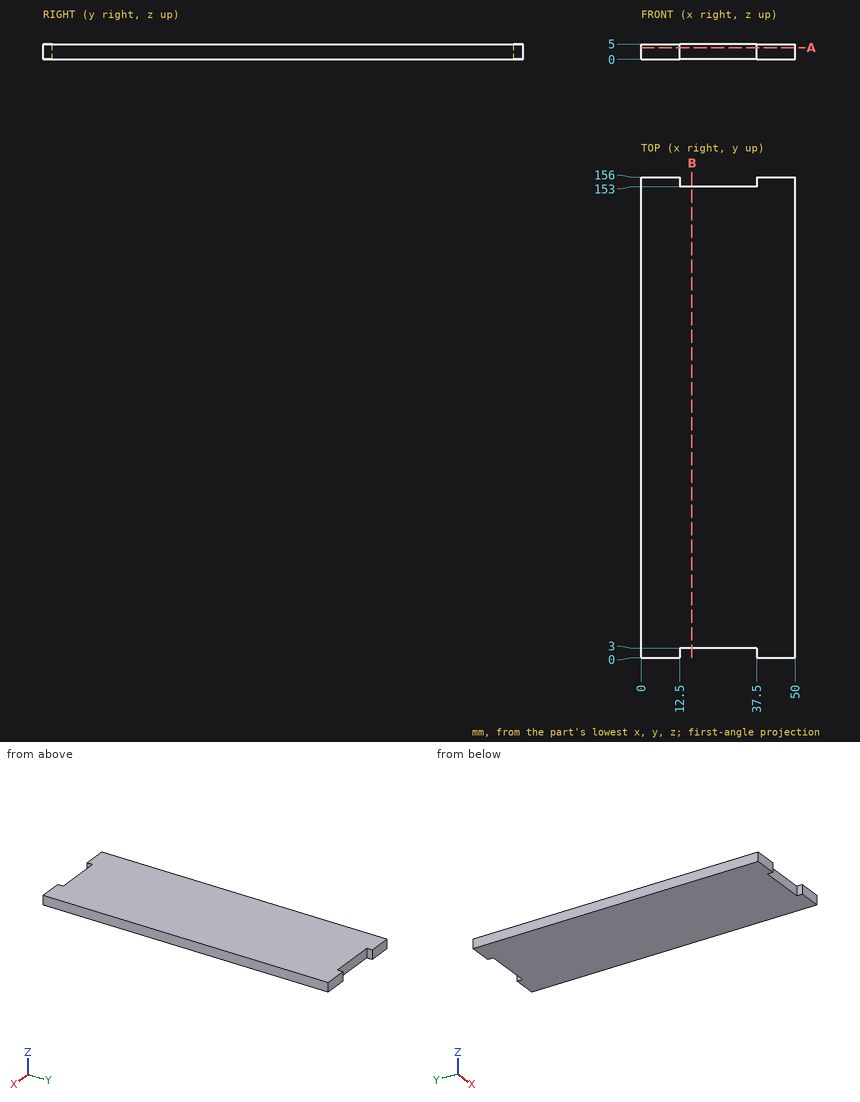
Study the drawing (mm; zero at the part's minimum x, y, z) and answer. Coordinates: 2 decimals unless noted, no trailing zeros. Write each loop counter-clockwise with the first axis right and the second up, starting at its lowest first coordinate (ties: lowest second). Pieces come first, ordered by that corner, then holes. Notation, with made-up numbers: (72, 30.25) - (93, 30.25) arc R12 ccw to (93, 40.25) - close; hole circle Ø6 at (83.25, 30). An arc over 180 degrees is marked (long way). Answer as a JSON object with one key per item and string values. Group by question number.
1. Consider L1, parallel to Y at x = 17, z = 1.2. Determine where the line is inside the solid, lowest interval first. Write a range as [from, to].
2. A cutting plane is placed at A-A (z = 3.85). Determine the outline of the cut face in (x, y).
3. A cutting plane is placed at B-B (x = 16.5). Determine the outline of the cut face in (y, z).
4. Each of these flat-tipped pins is pushed along its axis until it touches: P1, Ø1.5, axis at x = 21.5, z = 4.5, coming from the +Y side; P2, Ø2.5, axis at x = 25.5, z = 1.5, coming from the -Y side. Where does it stop, or does it pass through?
Worked out:
{
 "1": {"L1": "y = [3, 153]"},
 "2": {"outline": "(0, 0) - (12.5, 0) - (12.5, 3) - (37.5, 3) - (37.5, 0) - (50, 0) - (50, 156) - (37.5, 156) - (37.5, 153) - (12.5, 153) - (12.5, 156) - (0, 156) - close"},
 "3": {"outline": "(3, 0) - (153, 0) - (153, 5) - (3, 5) - close"},
 "4": {"P1": "stops at y = 153", "P2": "stops at y = 3"}
}
